Autodesk Inventor part; units mm, degrees
ref_plane "YZ Plane" through (0, 0, 0) normal (1, 0, 0) x (0, 1, 0)
ref_plane "XZ Plane" through (0, 0, 0) normal (0, 1, 0) x (-1, 0, 0)
ref_plane "XY Plane" through (0, 0, 0) normal (0, 0, 1) x (1, 0, 0)
sketch "スケッチ1" plane through (0, 0, 0) normal (0, 0, 1) x (1, 0, 0)
  line L0 (-20, -100) -> (20, -100)
  circle A0 centre (0, 0) radius 67.5
  dimension "d47" = 135
extrude "プレート1" add sketch "スケッチ1" along normal blind 4.5
sketch "スケッチ2" plane through (0, 0, 4.5) normal (0, 0, 1) x (1, 0, 0)
  circle A0 centre (0, 0) radius 62.5
  point P0 (-44.1942, -44.1942)
  point P1 (-16.1762, -60.3704)
  point P2 (16.1762, -60.3704)
  point P3 (44.1942, -44.1942)
  point P4 (60.3704, -16.1762)
  point P5 (60.3704, 16.1762)
  point P6 (44.1942, 44.1942)
  point P7 (16.1762, 60.3704)
  point P8 (-16.1762, 60.3704)
  point P9 (-44.1942, 44.1942)
  point P10 (-60.3704, 16.1762)
  point P11 (-60.3704, -16.1762)
  dimension "d5" = 125
  dimension "d8" = 360
  dimension "d51" = 0
hole "穴1" at (-60.3704, -16.1762, 4.5) at (-60.3704, 16.1762, 4.5) at (-44.1942, 44.1942, 4.5) at (-16.1762, 60.3704, 4.5) at (16.1762, 60.3704, 4.5) at (44.1942, 44.1942, 4.5) at (60.3704, 16.1762, 4.5) at (60.3704, -16.1762, 4.5) at (44.1942, -44.1942, 4.5) at (16.1762, -60.3704, 4.5) at (-16.1762, -60.3704, 4.5) at (-44.1942, -44.1942, 4.5) direction (0, 0, -1) diameter 4.3 end through all
sketch "スケッチ3" plane through (0, 0, 4.5) normal (0, 0, 1) x (1, 0, 0)
  circle A0 centre (0, 0) radius 27
  dimension "d18" = 54
extrude "押し出し1" cut sketch "スケッチ3" against normal blind 10
sketch "スケッチ4" plane through (0, 0, 4.5) normal (0, 0, 1) x (1, 0, 0)
  line L0 (10, -45) -> (-10, -45)
  line L1 (-10, -45) -> (-10, 45)
  line L2 (-10, 45) -> (10, 45)
  line L3 (10, 45) -> (10, -45)
  line L4 (10, -45) -> (-10, 45) construction
  line L5 (-10, -45) -> (10, 45) construction
  circle A0 centre (0, 0) radius 45.5
  point P0 (0, 0)
  point P1 (0, 0)
  dimension "d21" = 20
  dimension "d46" = 91
  dimension "d48" = 90
hole "穴2" at (-10, 45, 4.5) at (10, 45, 4.5) at (-10, -45, 4.5) at (10, -45, 4.5) direction (0, 0, -1) diameter 5.3 end through all
sketch "スケッチ5" plane through (0, 0, 4.5) normal (0, 0, 1) x (1, 0, 0)
  circle A0 centre (0, 0) radius 32
  point P0 (0, 32)
  point P1 (-27.7128, 16)
  point P2 (-27.7128, -16)
  point P3 (0, -32)
  point P4 (27.7128, -16)
  point P5 (27.7128, 16)
  dimension "d33" = 64
  dimension "d36" = 360
  dimension "d49" = 0
hole "穴3" at (0, 32, 4.5) at (-27.7128, 16, 4.5) at (-27.7128, -16, 4.5) at (0, -32, 4.5) at (27.7128, -16, 4.5) at (27.7128, 16, 4.5) direction (0, 0, -1) diameter 4.3 end through all
equation "\"d16\" = Thickness"
equation "\"d44\" = Thickness"
equation "\"d3\" = Thickness"
equation "\"BendRadius\" = Thickness"
equation "\"BendReliefWidth\" = Thickness"
equation "\"BendReliefDepth\" = 0.5 * Thickness"
equation "\"CornerReliefSize\" = 4 * Thickness"
equation "\"MinimumRemnant\" = 2 * Thickness"
equation "\"TransitionRadius\" = BendRadius"
equation "\"JacobiRadiusSize\" = BendRadius"
equation "\"GapSize\" = Thickness"
properties part number "scara-plate1" material "鋼、炭素鋼"
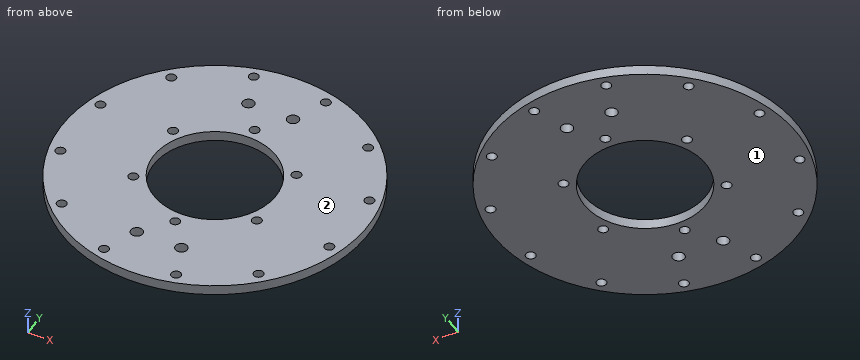
Geometry: final body of the model. Coordinates: model frame, mm. Face numbers are marked on the shaded views. Give positions to 0.01 mm unless a question says otherwise; leave off trailing zeros. Order: outer loops, then holes, each group sorted by start corner. A loop starts at its lowest first (then second) coordinate and runs counter-clockwise, first axis right, second up. Notation, with made-up numbers: (68, -33) -> (86, -33) arc R12 cw to (86, -22) -> close; hole circle Ø9 at (35, 59). An arc over 180 degrees is marked (long way). Put each result on its own line as item: value.
Q1. Pin query (flat end, axial travel): pin 1 (1 mm diameter, centred on x = -14, z = 4, fed in from -Y); pin 2 (5 mm diameter, centred on x = -16.18, y = 60.37, fed in from +Z); pin 3 (1 mm diameter, centred on y = 19, z = 2.5, fed in from -X); pin 4 (2 mm diameter, centred on y = 7, z = 1, fed in from -X). Return the tip coordinate at first contact, or that it passes through.
Here are the results:
pin 1: stops at y = -66.14
pin 2: stops at z = 4.5
pin 3: stops at x = -64.92
pin 4: stops at x = -67.23
Q2. Section B-B, the plane x = -4.5. Return loops of the section in (y, z).
Here are the results:
outline: (-67.35, 0) -> (-26.62, 0) -> (-26.62, 4.5) -> (-67.35, 4.5) -> close; (26.62, 0) -> (67.35, 0) -> (67.35, 4.5) -> (26.62, 4.5) -> close
Q3. Section D-D, the plane y = 16. Return loops of the section in (x, z).
Here are the results:
outline: (-65.58, 0) -> (-62.51, 0) -> (-62.51, 4.5) -> (-65.58, 4.5) -> close; (-58.23, 0) -> (-29.86, 0) -> (-29.86, 4.5) -> (-58.23, 4.5) -> close; (-25.56, 0) -> (-21.75, 0) -> (-21.75, 4.5) -> (-25.56, 4.5) -> close; (21.75, 0) -> (25.56, 0) -> (25.56, 4.5) -> (21.75, 4.5) -> close; (29.86, 0) -> (58.23, 0) -> (58.23, 4.5) -> (29.86, 4.5) -> close; (62.51, 0) -> (65.58, 0) -> (65.58, 4.5) -> (62.51, 4.5) -> close
Q4. Section C-C, the plane z = 3.35. Count the separate pieces of the cut face and the enclosed holes in it, then the cut area to 3 significant figures.
Here are the results:
separate pieces: 1
enclosed holes: 23
area: 11,700 mm^2
Q5. Section A-A, the plane y = -2.5. Return loops of the section in (x, z), then the cut area to 3 significant figures.
Here are the results:
outline: (-67.45, 0) -> (-26.88, 0) -> (-26.88, 4.5) -> (-67.45, 4.5) -> close; (26.88, 0) -> (67.45, 0) -> (67.45, 4.5) -> (26.88, 4.5) -> close
area: 365 mm^2
Q6. Material intervals for L1, parallel to Y at x = 17.5, z = 1.7; L2, parallel to Y at x = -16, z = 0.85; L3, parallel to Y at x = -29, z = 2.45, sorted ascending.
Here are the results:
L1: y = -65.19 to -62.06, -58.68 to -20.56, 20.56 to 58.68, 62.06 to 65.19
L2: y = -65.58 to -62.51, -58.23 to -21.75, 21.75 to 58.23, 62.51 to 65.58
L3: y = -60.95 to -17.72, -14.28 to 14.28, 17.72 to 60.95
Q7. Draft query along Z for the marked faces 1 and 2. Return one class per face: released by +Z, released by -Z, zero draft, split by the parting line, or undercut.
Here are the results:
face 1: released by -Z
face 2: released by +Z
